Here's the drawing with two shaded views (mm, measured from the low corner). I have some questions. A direction names the side the tool comes from. Coordinates: 2 decimals unless noted, no trailing zeros. Order: outer loops, then holes, each group sorted by start corner. A loop starts at its lowest first (then second) coordinate and runs counter-clockwise, first axis right, second up. Notation, with made-up numbers: (54, 2) -> (97, 2) arc R22 cw to (97, 38) -> close; hole circle Ø6 at (-34, -17). An arc over 180 degrees is marked (long way). One line per item, written item: value. Start each with the question number.
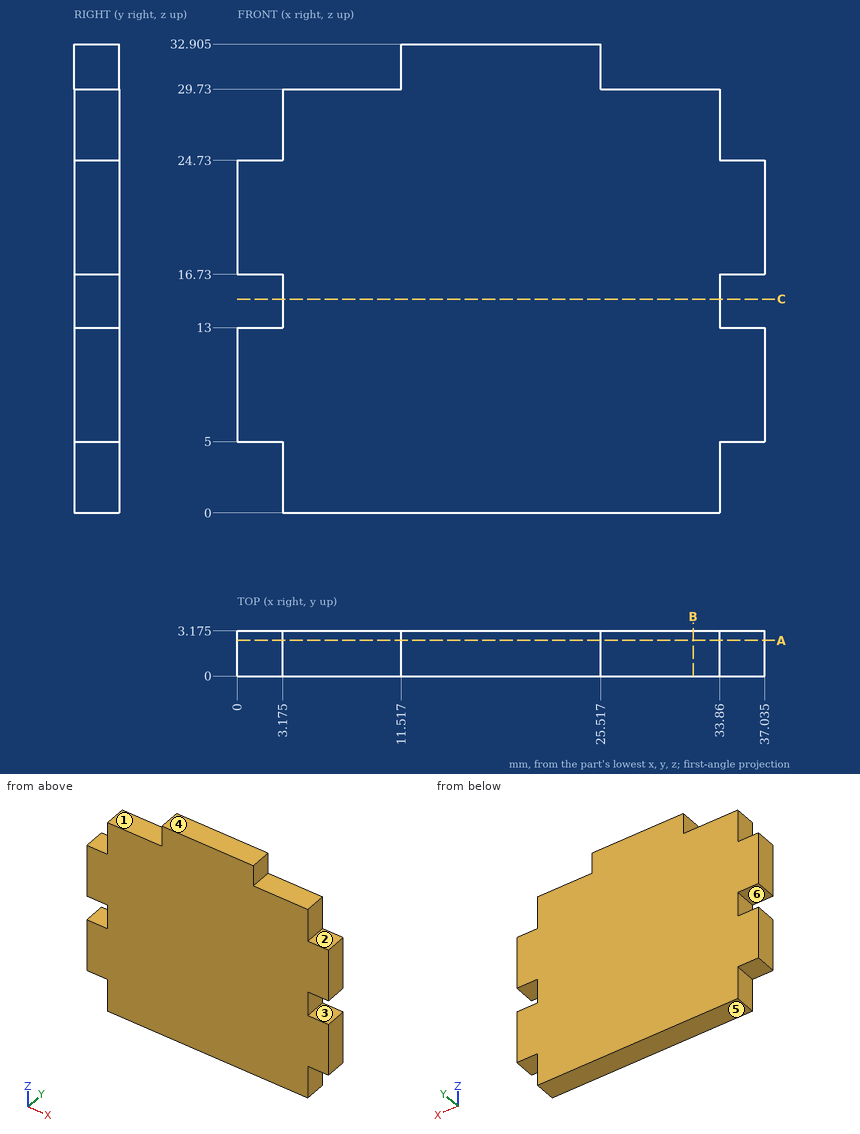
Q1. If we mould it in two halves opening along Z, with no side actions, what happens to the marked faces 4, 5 and 6? For each: +Z half, -Z half, draft (parallel to the pull), parting line (faces both ways), or undercut.
Q2. Imagine slicing it at C-C (z = 15). Write out the boundary of the cut face in (x, y) (1 decimal).
Q3. Imagine slicing it at B-B (x = 32). Write out the boundary of the cut face in (y, z) (1 decimal).
Q4. For P1, Ø10, axis at x = 10, z = 20, coming from the -Y side; P2, Ø1, axis at x = 36, y = 2, coming from the +Z side; P3, Ø1.6, axis at x = 1.5, y = 2.5, coming from the -Z side; P4, Ø1.6, axis at y = 2, z = 1.5, coming from the -X side (3 decimals), each with a flat end and sliding along its axis, tell me the tip position at first contact or that it passes through.
Q5. For the marked faces 1, 2 and 3, which set-ups out of +Z, -Z, +X, -X, +Y, -Y let a thin tool reach every point of the face, with its end or its side?
Q6. I need wall thicknesses on line 1 (Z direction, x = 35.5, y = 2.85); line 2 (Z direction, x = 6.5, y = 2.6); line 3 (X direction, y = 2, z = 4.5) (1 decimal). Which ranges of each line are inside material? Lowest first, please.
Q7. Imagine slicing it at A-A (y = 2.5). Write out the boundary of the cut face in (x, z) (1 decimal).
Completed:
1. face 4: +Z half
1. face 5: -Z half
1. face 6: undercut
2. outline: (3.2, 0) -> (33.9, 0) -> (33.9, 3.2) -> (3.2, 3.2) -> close
3. outline: (0, 0) -> (3.2, 0) -> (3.2, 29.7) -> (0, 29.7) -> close
4. P1: stops at y = 0
4. P2: stops at z = 24.73
4. P3: stops at z = 5
4. P4: stops at x = 3.175
5. face 1: +Z, -X, +Y, -Y
5. face 2: +Z, +X, +Y, -Y
5. face 3: +X, +Y, -Y
6. line 1: z = 5 to 13, 16.73 to 24.73
6. line 2: z = 0 to 29.73
6. line 3: x = 3.2 to 33.9
7. outline: (0, 5) -> (3.2, 5) -> (3.2, 0) -> (33.9, 0) -> (33.9, 5) -> (37, 5) -> (37, 13) -> (33.9, 13) -> (33.9, 16.7) -> (37, 16.7) -> (37, 24.7) -> (33.9, 24.7) -> (33.9, 29.7) -> (25.5, 29.7) -> (25.5, 32.9) -> (11.5, 32.9) -> (11.5, 29.7) -> (3.2, 29.7) -> (3.2, 24.7) -> (0, 24.7) -> (0, 16.7) -> (3.2, 16.7) -> (3.2, 13) -> (0, 13) -> close
